from build123d import *

# Parameters (mm, degrees)
SKETCH_1_W                = 220
SKETCH_1_H                = 165
EXTRUDE_1_DEPTH           = 166
FILLET_1_R                = 3
SKETCH_2_W                = 232
SKETCH_2_H                = 175
EXTRUDE_2_DEPTH           = 30
FILLET_2_R                = 2
SKETCH_3_R                = 14
EXTRUDE_3_DEPTH           = 3.6
SKETCH_5_R                = 8.8
EXTRUDE_4_DEPTH           = 18.5
EXTRUDE_4_DRAFT           = 2
EXTRUDE_4_PROFILE_2_DEPTH = 18.5
EXTRUDE_4_PROFILE_2_DRAFT = 2


with BuildPart() as part:
    # Эскиз1 → Вытянуть1 (new body)
    with BuildSketch(Plane(origin=(0, 0, 0), x_dir=(1, 0, 0), z_dir=(0, 1, 0))):
        Rectangle(SKETCH_1_W, SKETCH_1_H)
    extrude(amount=EXTRUDE_1_DEPTH)

    # Скругление1
    fillet_1_edges = [part.edges().sort_by_distance(p)[0] for p in [
        (110, 83, 82.5),
        (-110, 83, 82.5),
        (-110, 83, -82.5),
        (110, 83, -82.5),
    ]]
    fillet(fillet_1_edges, radius=FILLET_1_R)

    # Эскиз2 → Вытянуть2 (add)
    with BuildSketch(Plane(origin=(0, 166, 0), x_dir=(1, 0, 0), z_dir=(0, 1, 0))):
        Rectangle(SKETCH_2_W, SKETCH_2_H)
    extrude(amount=EXTRUDE_2_DEPTH)

    # Скругление2
    fillet_2_edges = [part.edges().sort_by_distance(p)[0] for p in [
        (116, 166, 0),
        (116, 181, 87.5),
        (0, 166, -87.5),
        (116, 181, -87.5),
        (-116, 166, 0),
        (-116, 181, -87.5),
        (0, 166, 87.5),
        (-116, 181, 87.5),
        (116, 196, 0),
        (0, 196, -87.5),
        (-116, 196, 0),
        (0, 196, 87.5),
    ]]
    fillet(fillet_2_edges, radius=FILLET_2_R)

    # Эскиз3 → Вытянуть3 (add)
    with BuildSketch(Plane(origin=(0, 196, 0), x_dir=(1, 0, 0), z_dir=(0, 1, 0))):
        with Locations(Location((96, -47.5, 0), (0, 0, 270))):
            Circle(SKETCH_3_R)
        with Locations(Location((-96, -47.5, 0), (0, 0, 90))):
            Circle(SKETCH_3_R)
    extrude(amount=EXTRUDE_3_DEPTH)


with BuildPart() as extrude_4_tool:
    # Эскиз5 → Вытянуть4 (with draft: the straight prism first)
    with BuildSketch(Plane(origin=(0, 199.6, 0), x_dir=(1, 0, 0), z_dir=(0, 1, 0))):
        with Locations((96, -47.5)):
            Circle(SKETCH_5_R)
    extrude(amount=EXTRUDE_4_DEPTH)
    # Вытянуть4: the draft: its side faces are tilted about the plane it starts from
    extrude_4_sides = [extrude_4_tool.faces().sort_by_distance(p)[0] for p in [
        (87.2, 208.85, 47.5),
    ]]
    draft(extrude_4_sides, Plane(origin=(0, 199.6, 0), x_dir=(1, 0, 0), z_dir=(0, 1, 0)), EXTRUDE_4_DRAFT)


with BuildPart() as part_1:
    add(part.part)

    # Вытянуть4: add extrude_4_tool
    add(extrude_4_tool.part)


with BuildPart() as extrude_4_profile_2_tool:
    # Эскиз5 → Вытянуть4 profile 2 (with draft: the straight prism first)
    with BuildSketch(Plane(origin=(0, 199.6, 0), x_dir=(1, 0, 0), z_dir=(0, 1, 0))):
        with Locations((-96, -47.5)):
            Circle(SKETCH_5_R)
    extrude(amount=EXTRUDE_4_PROFILE_2_DEPTH)
    # Вытянуть4 profile 2: the draft: its side faces are tilted about the plane it starts from
    extrude_4_profile_2_sides = [extrude_4_profile_2_tool.faces().sort_by_distance(p)[0] for p in [
        (-104.8, 208.85, 47.5),
    ]]
    draft(extrude_4_profile_2_sides, Plane(origin=(0, 199.6, 0), x_dir=(1, 0, 0), z_dir=(0, 1, 0)), EXTRUDE_4_PROFILE_2_DRAFT)


with BuildPart() as part_2:
    add(part_1.part)

    # Вытянуть4 profile 2: add extrude_4_profile_2_tool
    add(extrude_4_profile_2_tool.part)


solid = part_2.part
Work out the finished part from the listing and answer in its coordinate system (mm). A direction names the side the tool comes from. Coordinates: 2 decimals unless noted, no trailing zeros. Order: outer loops, then holes, each group sorted by start corner. A loop starts at its lowest first (then second) coordinate and runs counter-clockwise, first axis right, second up. Notation, with made-up numbers: (15, -11.75) - (69, -11.75) arc R8 cw to (69, -0.75) - close; hole circle Ø7 at (-21.75, -9). An arc over 180 degrees is marked (long way). Put each result on its own line as item: value. Start each with the question number.
1) Find the intervals of material crossed by line 1 (Z direction, x = 56, y = 26); line 2 (X direction, y = 13, z = 7.5); line 3 (Y direction, x = -55, z = -63.5), in increasing order. Write a range as from..to.
2) Find section B-B (y = 149). Give the vertices of the cut face in (x, z).
3) For faces 5 (the flat face through (96, 199.6, 57)), 6 (the flat face through (-110, 82, 1)), 7 (the flat face through (-1, 82, -82.5)), determine the directions among +Z, -Z, +X, -X, +Y, -Y from which every point of the face is accessible in a straight line to the end or side of a thin tool.
4) For a pull along X with two mould halves and no side action, classify faces 1 (the flat face through (-96, 199.6, 38)), 2 (the cylindrical face through (109.88, 197.77, 45.68)), 3 (the flat face through (-1, 82, 82.5)), 4 (the flat face through (110, 82, 1)) as released by +X, released by -X, zero draft, split by the parting line, or undercut.
5) Flat-ended cylindrical pins translate along their axes: pin 1 (5 mm diameter, centred on x = -91.5, y = 72.5, fed in from +Z); pin 2 (4 mm diameter, centred on x = 77, y = 123.5, fed in from -Z); pin 3 (4 mm diameter, centred on x = -70.5, z = 52.5, fed in from +Y). Find the tip coordinate at first contact, or state that the pin passes through.
6) Find section D-D (z = -19). Give the vertices of the cut face in (x, y).
7) Find section A-A (z = 47.5). Give the vertices of the cut face in (x, y), plus the area to 3 significant figures.
8) Find section C-C (x = 21). Give the vertices of the cut face in (y, z).
Results list:
1. line 1: z = -82.5..82.5
1. line 2: x = -110..110
1. line 3: y = 0..196
2. outline: (-110, -79.5) arc R3 ccw to (-107, -82.5) - (107, -82.5) arc R3 ccw to (110, -79.5) - (110, 79.5) arc R3 ccw to (107, 82.5) - (-107, 82.5) arc R3 ccw to (-110, 79.5) - close
3. face 5: +Y
3. face 6: +Z, -Z, -X, -Y
3. face 7: -Z, +X, -X, -Y
4. face 1: undercut
4. face 2: undercut
4. face 3: zero draft
4. face 4: released by +X
5. pin 1: stops at z = 82.5
5. pin 2: stops at z = -82.5
5. pin 3: stops at y = 196
6. outline: (-116, 168) arc R2 ccw to (-114, 166) - (-110, 166) - (-110, 0) - (110, 0) - (110, 166) - (114, 166) arc R2 ccw to (116, 168) - (116, 194) arc R2 ccw to (114, 196) - (-114, 196) arc R2 ccw to (-116, 194) - close
7. outline: (-116, 168) arc R2 ccw to (-114, 166) - (-110, 166) - (-110, 0) - (110, 0) - (110, 166) - (114, 166) arc R2 ccw to (116, 168) - (116, 194) arc R2 ccw to (114, 196) - (110, 196) - (110, 199.6) - (104.8, 199.6) - (104.15, 218.1) - (87.85, 218.1) - (87.2, 199.6) - (82, 199.6) - (82, 196) - (-82, 196) - (-82, 199.6) - (-87.2, 199.6) - (-87.85, 218.1) - (-104.15, 218.1) - (-104.8, 199.6) - (-110, 199.6) - (-110, 196) - (-114, 196) arc R2 ccw to (-116, 194) - close
7. area: 44,300 mm^2
8. outline: (0, -82.5) - (166, -82.5) - (166, -85.5) arc R2 ccw to (168, -87.5) - (194, -87.5) arc R2 ccw to (196, -85.5) - (196, 85.5) arc R2 ccw to (194, 87.5) - (168, 87.5) arc R2 ccw to (166, 85.5) - (166, 82.5) - (0, 82.5) - close
